Verification items for the finished model (mm, model axes). Face numbers are marked on the shaded views. A direction names the side the tool comes from. Round coordinates to 2 decimals unless told otherwise and drop trailing zeros. Write each loop counter-clockwise with the first axis right and the second up, starting at its lowest first coordinate (ties: lowest second). Pieces come first, ordered by that corner, then holes. Notation, with made-up numbers: (9, 0) - (45, 0) arc R22 cw to (45, 7) - close; hole circle Ø5 at (0.5, 4). An arc over 180 degrees is marked (long way). Write each question's results on one line, items separated by ' | '.
```python
from build123d import *

# Parameters (mm, degrees)
SKETCH1_R               = 14
SKETCH1_R_2             = 2.25
BOSS_EXTRUDE1_DEPTH     = 5
SKETCH2_R               = 1.5
CUT_EXTRUDE1_DEPTH      = 21.420577857
SKETCH4_R               = 3.5
CUT_EXTRUDE2_DEPTH      = 3
CIRPATTERN1_COUNT       = 2
SKETCH5_R               = 13
SKETCH5_R_2             = 8
BOSS_EXTRUDE2_DEPTH     = 7
SKETCH6_R               = 3.5
CUT_EXTRUDE3_DEPTH      = 22
CHAMFER1_SIZE           = 2
FILLET1_START           = 5
FILLET1_DEPTH           = 8
CUT_EXTRUDE4_DEPTH      = 24.151673806
CUT_EXTRUDE4_DEPTH_BACK = 24.151673806
SKETCH8_R               = 2.1
CHAMFER2_SIZE           = 2


with BuildPart() as part:
    # Sketch1 → Boss-Extrude1 (new body)
    with BuildSketch(Plane(origin=(0, 0, 0), x_dir=(1, 0, 0), z_dir=(0, 1, 0))):
        with Locations(Location((0, 0, 0), (0, 0, 270))):
            Circle(SKETCH1_R)
        with Locations(Location((0, 0, 0), (0, 0, 270))):
            Circle(SKETCH1_R_2, mode=Mode.SUBTRACT)
    extrude(amount=BOSS_EXTRUDE1_DEPTH)

    # Sketch2 → Cut-Extrude1 (cut, through all)
    with BuildSketch(Plane(origin=(0, 5, 0), x_dir=(1, 0, 0), z_dir=(0, 1, 0))):
        with Locations(Location((0, 9, 0), (0, 0, 270))):
            Circle(SKETCH2_R)
    cut_extrude1 = extrude(amount=-CUT_EXTRUDE1_DEPTH, mode=Mode.SUBTRACT)

    # Sketch4 → Cut-Extrude2 (cut)
    with BuildSketch(Plane(origin=(0, 5, 0), x_dir=(1, 0, 0), z_dir=(0, 1, 0))):
        with Locations(Location((0, 9, 0), (0, 0, 270))):
            Circle(SKETCH4_R)
    cut_extrude2 = extrude(amount=-CUT_EXTRUDE2_DEPTH, mode=Mode.SUBTRACT)

    # CirPattern1: Cut-Extrude1, Cut-Extrude2 ×2 about axis
    cirpattern1_axis = Axis((0, 0, 0), (0, 1, 0))
    add([cut_extrude1.rotate(cirpattern1_axis, i * 360 / CIRPATTERN1_COUNT) for i in range(1, CIRPATTERN1_COUNT)], mode=Mode.SUBTRACT)
    add([cut_extrude2.rotate(cirpattern1_axis, i * 360 / CIRPATTERN1_COUNT) for i in range(1, CIRPATTERN1_COUNT)], mode=Mode.SUBTRACT)

    # Sketch5 → Boss-Extrude2 (add)
    with BuildSketch(Plane(origin=(0, 5, 0), x_dir=(1, 0, 0), z_dir=(0, 1, 0))):
        with Locations(Location((0, 0, 0), (0, 0, 270))):
            Circle(SKETCH5_R)
        with Locations(Location((0, 0, 0), (0, 0, 112.7982481))):
            Circle(SKETCH5_R_2, mode=Mode.SUBTRACT)
    extrude(amount=BOSS_EXTRUDE2_DEPTH)

    # Sketch6 → Cut-Extrude3 (cut, through all)
    with BuildSketch(Plane(origin=(0, 5, 0), x_dir=(1, 0, 0), z_dir=(0, 1, 0))):
        with Locations(Location((0, 9, 0), (0, 0, 270))):
            Circle(SKETCH6_R)
        with Locations(Location((0, -9, 0), (0, 0, 27.664004496))):
            Circle(SKETCH6_R)
    extrude(amount=CUT_EXTRUDE3_DEPTH, mode=Mode.SUBTRACT)

    # Chamfer1
    # the kernel refuses this chamfer: 2 mm, written as the material it adds along each edge
    with BuildSketch(Plane(origin=(0, 5, 0), x_dir=(0, 0, 1), z_dir=(-1, 0, 0))) as chamfer1_piece_1_section:
        Polygon((13 + CHAMFER1_SIZE, 0), (13, CHAMFER1_SIZE), (13, 0), align=None)
    chamfer1_piece_1 = revolve(axis=Axis((0, 5, 0), (0, 1, 0)), mode=Mode.PRIVATE)
    chamfer1_piece_1 = chamfer1_piece_1 & Plane(origin=(0, 5, 0), x_dir=(0, 0, 1), z_dir=(0, -1, 0)) * Cylinder(14, 61, mode=Mode.PRIVATE)
    add(chamfer1_piece_1)

    # Fillet1: read off the stored shape, not the designer's step
    # Fillet1 outline → Fillet1 (cut)
    with BuildSketch(Plane(origin=(0, 0, 0), x_dir=(1, 0, 0), z_dir=(0, 1, 0)).offset(FILLET1_START)):
        with BuildLine():
            ThreePointArc((3.388860428, -8.125), (3.438547611, -7.479715292), (3.872983346, -7))
            ThreePointArc((3.872983346, -7), (3.491479482, -7.197886567), (3.099899192, -7.375))
            ThreePointArc((3.099899192, -7.375), (3.265979999, -7.741677844), (3.388860428, -8.125))
        make_face()
        with BuildLine():
            ThreePointArc((3.099899192, 7.375), (3.491479482, 7.197886567), (3.872983346, 7))
            ThreePointArc((3.872983346, 7), (3.438547611, 7.479715292), (3.388860428, 8.125))
            ThreePointArc((3.388860428, 8.125), (3.265979999, 7.741677844), (3.099899192, 7.375))
        make_face()
        with BuildLine():
            ThreePointArc((-3.388860428, -8.125), (-3.265979999, -7.741677844), (-3.099899192, -7.375))
            ThreePointArc((-3.099899192, -7.375), (-3.491479482, -7.197886567), (-3.872983346, -7))
            ThreePointArc((-3.872983346, -7), (-3.438547611, -7.479715292), (-3.388860428, -8.125))
        make_face()
        with BuildLine():
            ThreePointArc((-3.872983346, 7), (-3.491479482, 7.197886567), (-3.099899192, 7.375))
            ThreePointArc((-3.099899192, 7.375), (-3.265979999, 7.741677844), (-3.388860428, 8.125))
            ThreePointArc((-3.388860428, 8.125), (-3.438547611, 7.479715292), (-3.872983346, 7))
        make_face()
    extrude(amount=FILLET1_DEPTH, mode=Mode.SUBTRACT)

    # Sketch8 → Cut-Extrude4 (cut, two sides: drawn at the far end of the back side and taken through both)
    with BuildSketch(Plane(origin=(0, 0, 0), x_dir=(0, 0, -1), z_dir=(1, 0, 0)).offset(-CUT_EXTRUDE4_DEPTH_BACK)):
        with Locations((0, 8.75)):
            Circle(SKETCH8_R)
    extrude(amount=CUT_EXTRUDE4_DEPTH + CUT_EXTRUDE4_DEPTH_BACK, mode=Mode.SUBTRACT)

    # Chamfer2
    # the kernel refuses this chamfer: 2 mm, written as the material it takes off along each edge
    with BuildSketch(Plane(origin=(0, 12, 0), x_dir=(0, 0, 1), z_dir=(-1, 0, 0))) as chamfer2_piece_1:
        Polygon((13, -CHAMFER2_SIZE), (13 - CHAMFER2_SIZE, 0), (13, 0), align=None)
    revolve(axis=Axis((0, 12, 0), (0, 1, 0)), mode=Mode.SUBTRACT)


solid = part.part
```
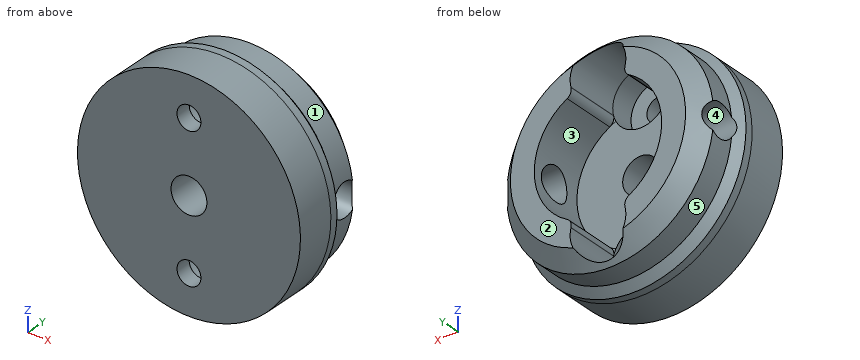
(1) Set-up check for the marked faces 1 and 2: record each of +Z, -Z, +X, -X, +Y, -Y from which the full face is reachable in a straight line by a thin tool's end or side.
Answer:
face 1: +Z, +Y | face 2: +Z, -Z, +X, -X, +Y
(2) Section check C-C (y = 8.75). Record the cut outline in (x, z) (3 decimals), plus the area to 3 significant figures.
Answer:
outline: (-12.829, -2.1) arc R13 ccw to (12.829, -2.1) - (7.719, -2.1) arc R8 cw to (3.873, -7) arc R1 ccw to (3.389, -8.125) arc R3.5 cw (long way) to (-3.389, -8.125) arc R1 ccw to (-3.873, -7) arc R8 cw to (-7.719, -2.1) - close; (-12.829, 2.1) - (-7.719, 2.1) arc R8 cw to (-3.873, 7) arc R1 ccw to (-3.389, 8.125) arc R3.5 cw (long way) to (3.389, 8.125) arc R1 ccw to (3.873, 7) arc R8 cw to (7.719, 2.1) - (12.829, 2.1) arc R13 ccw to start | area: 232 mm2
(3) Mould release check, pull along X, two halves, no side actions. Record for the marked faces 3, 4 and 5: released by +X, released by -X, zero draft, split by the parting line, or undercut.
Answer:
face 3: undercut | face 4: zero draft | face 5: split by the parting line
(4) Section check A-A (z = 0). Record the cut outline in (x, y).
Answer:
outline: (-14, 0) - (-2.25, 0) - (-2.25, 5) - (-8, 5) - (-8, 6.65) - (-13.35, 6.65) - (-14, 6) - close; (-12.15, 10.85) - (-8, 10.85) - (-8, 12) - (-11, 12) - close; (2.25, 0) - (14, 0) - (14, 6) - (13.35, 6.65) - (8, 6.65) - (8, 5) - (2.25, 5) - close; (8, 10.85) - (12.15, 10.85) - (11, 12) - (8, 12) - close
(5) Go/stop test with flat-tipped pins: pin 1 Ø4 at (x, z) = (0, 0) entering from +Y; pin 2 Ø4 at (x, z) = (0, 9) entering from +Y; pin 3 Ø4 at (y, z) = (2.5, 5.5) entering from -X; pin 4 Ø3 at (x, y) = (6.5, 1.5) entering from +Z. Record where each tip stops, or that it passes through.
Answer:
pin 1: through | pin 2: y = 2 | pin 3: x = -13.56 | pin 4: z = 13.08
(6) Thickness scan on L1, parallel to X at y = 2.6, z = 0; L2, parallel to Z at x = 0, y = 10; L3, parallel to X at y = 1.3, z = 9. Record the ranges inside material, lowest first.
Answer:
L1: -14 to -2.25, 2.25 to 14 | L2: -13 to -12.5, 12.5 to 13 | L3: -10.72 to -1.5, 1.5 to 10.72
(7) Section check B-B (x = 0). Record the cut outline in (y, z).
Answer:
outline: (0, -14) - (6, -14) - (7, -13) - (10, -13) - (10.5, -12.5) - (2, -12.5) - (2, -10.5) - (0, -10.5) - close; (0, -7.5) - (2, -7.5) - (2, -5.5) - (5, -5.5) - (5, -2.25) - (0, -2.25) - close; (0, 2.25) - (5, 2.25) - (5, 5.5) - (2, 5.5) - (2, 7.5) - (0, 7.5) - close; (0, 10.5) - (2, 10.5) - (2, 12.5) - (10.5, 12.5) - (10, 13) - (7, 13) - (6, 14) - (0, 14) - close
